Geometry: see drawing. Coordinates: mm, zero at the bounding-box minimum. Coordinates: 2 decimals unless noted, no trailing zeros. Write each loop counter-clockwise with the first axis right and the second up, starting at its lowest first coordinate (ties: lowest second). Pieces come first, ordered by that corner, then holes. Notation, with made-up numbers: (-11.75, 21) - (18.25, 21) arc R12 cw to (18.25, 26) - close; hole circle Ø2 at (-12.75, -12.75). An arc over 180 degrees is marked (long way). Use a Markdown table: item, result. Add a question column.
Q1. Material intervals for probe 1 along Z at (x, y) = (26, 0.2); probe 2 along Y at (x, z) = (12, 52.5); probe 3 along X at (y, z) = (2.85, 30.5), sorted ascending. Write a range as from..to.
Q2. Section query A-A (y = 0.85). Return the cut outline in (x, z).
Q3. Section query B-B (x = 45). Return the cut outline in (y, z).
Q4. Section query C-C (z = 24.5). Return the cut outline in (x, y).
Q5. Pin query (flat end, axial travel): P1, Ø1.5, axis at y = 1.5, z = 3, coming from the -X side; P2, Ø0.9, axis at y = 1, z = 1.5, coming from the +X side; P3, Ø3, axis at x = 9, z = 26, coming from the -Y side. Return the tip coordinate at first contact, or that it passes through.
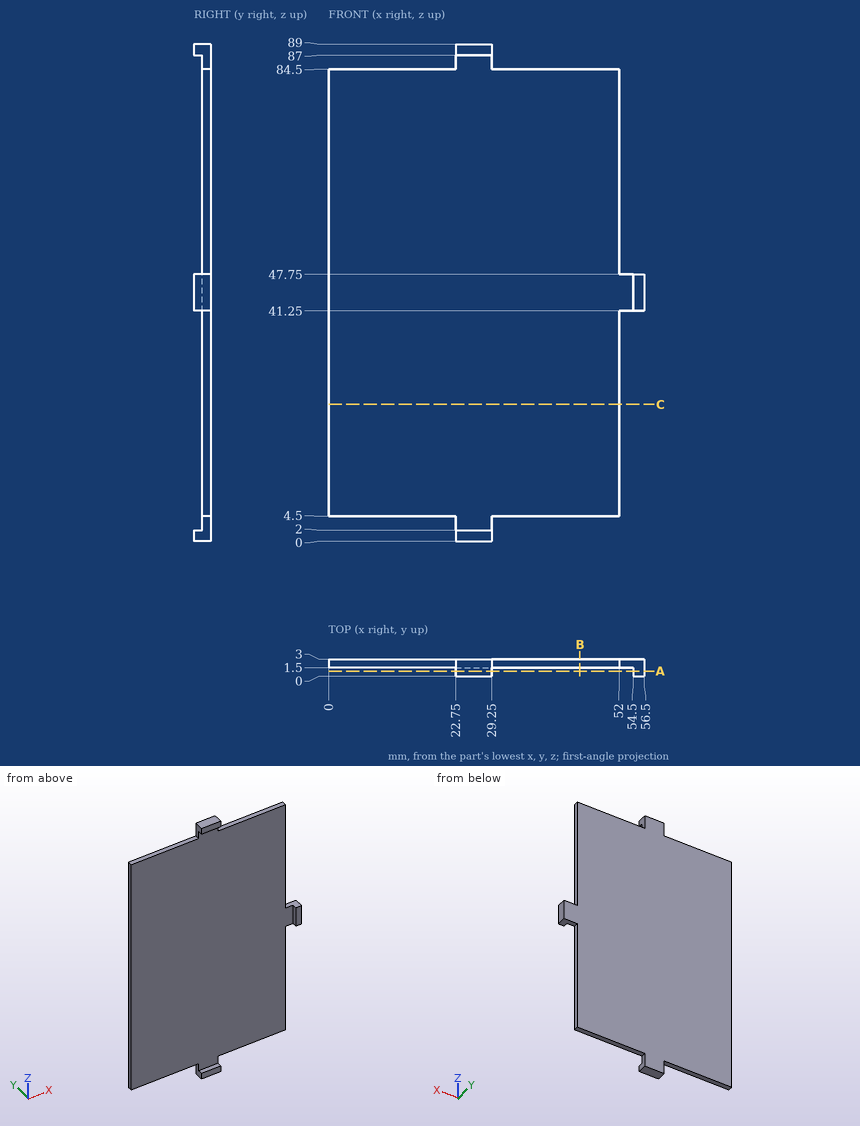
Values follow:
| question | item | result |
|---|---|---|
| 1 | probe 1 | 0..2, 87..89 |
| 1 | probe 2 | 1.5..3 |
| 1 | probe 3 | 0..52 |
| 2 | outline | (22.75, 0) - (29.25, 0) - (29.25, 2) - (22.75, 2) - close; (22.75, 87) - (29.25, 87) - (29.25, 89) - (22.75, 89) - close; (54.5, 41.25) - (56.5, 41.25) - (56.5, 47.75) - (54.5, 47.75) - close |
| 3 | outline | (1.5, 4.5) - (3, 4.5) - (3, 84.5) - (1.5, 84.5) - close |
| 4 | outline | (0, 1.5) - (52, 1.5) - (52, 3) - (0, 3) - close |
| 5 | P1 | x = 22.75 |
| 5 | P2 | x = 29.25 |
| 5 | P3 | y = 1.5 |
